from build123d import *

# Parameters (mm, degrees)
CROQUIS1_R              = 3.4
SALIENTE_EXTRUIR1_DEPTH = 360


with BuildPart() as part:
    # Croquis1 → Saliente-Extruir1 (new body)
    with BuildSketch(Plane.XY):
        with BuildLine():
            Line((-4.433640906, 1.227432273), (-4.433640906, 9.707432273))
            Line((-4.433640906, 9.707432273), (1.236359094, 15.377432273))
            Line((1.236359094, 15.377432273), (4.426359094, 15.377432273))
            Line((4.426359094, 15.377432273), (4.426359094, 11.197432273))
            Line((4.426359094, 11.197432273), (5.426359094, 11.197432273))
            ThreePointArc((5.426359094, 11.197432273), (6.133465875, 11.490325492), (6.426359094, 12.197432273))
            Line((6.426359094, 12.197432273), (6.426359094, 19.627432273))
            ThreePointArc((6.426359094, 19.627432273), (5.694126047, 21.395199226), (3.926359094, 22.127432273))
            Line((3.926359094, 22.127432273), (-3.503640906, 22.127432273))
            ThreePointArc((-3.503640906, 22.127432273), (-4.210747688, 21.834539054), (-4.503640906, 21.127432273))
            Line((-4.503640906, 21.127432273), (-4.503640906, 20.127432273))
            Line((-4.503640906, 20.127432273), (-0.323640906, 20.127432273))
            Line((-0.323640906, 20.127432273), (-0.323640906, 16.937432273))
            Line((-0.323640906, 16.937432273), (-5.993640906, 11.267432273))
            Line((-5.993640906, 11.267432273), (-14.473640906, 11.267432273))
            Line((-14.473640906, 11.267432273), (-20.143640906, 16.937432273))
            Line((-20.143640906, 16.937432273), (-20.143640906, 20.127432273))
            Line((-20.143640906, 20.127432273), (-15.963640906, 20.127432273))
            Line((-15.963640906, 20.127432273), (-15.963640906, 21.127432273))
            ThreePointArc((-15.963640906, 21.127432273), (-16.256534125, 21.834539054), (-16.963640906, 22.127432273))
            Line((-16.963640906, 22.127432273), (-24.393640906, 22.127432273))
            ThreePointArc((-24.393640906, 22.127432273), (-26.161407859, 21.395199226), (-26.893640906, 19.627432273))
            Line((-26.893640906, 19.627432273), (-26.893640906, 12.197432273))
            ThreePointArc((-26.893640906, 12.197432273), (-26.600747688, 11.490325492), (-25.893640906, 11.197432273))
            Line((-25.893640906, 11.197432273), (-24.893640906, 11.197432273))
            Line((-24.893640906, 11.197432273), (-24.893640906, 15.377432273))
            Line((-24.893640906, 15.377432273), (-21.703640906, 15.377432273))
            Line((-21.703640906, 15.377432273), (-16.033640906, 9.707432273))
            Line((-16.033640906, 9.707432273), (-16.033640906, 1.227432273))
            Line((-16.033640906, 1.227432273), (-21.703640906, -4.442567727))
            Line((-21.703640906, -4.442567727), (-24.893640906, -4.442567727))
            Line((-24.893640906, -4.442567727), (-24.893640906, -0.262567727))
            Line((-24.893640906, -0.262567727), (-25.893640906, -0.262567727))
            ThreePointArc((-25.893640906, -0.262567727), (-26.600747688, -0.555460946), (-26.893640906, -1.262567727))
            Line((-26.893640906, -1.262567727), (-26.893640906, -8.692567727))
            ThreePointArc((-26.893640906, -8.692567727), (-26.161407859, -10.46033468), (-24.393640906, -11.192567727))
            Line((-24.393640906, -11.192567727), (-16.963640906, -11.192567727))
            ThreePointArc((-16.963640906, -11.192567727), (-16.256534125, -10.899674508), (-15.963640906, -10.192567727))
            Line((-15.963640906, -10.192567727), (-15.963640906, -9.192567727))
            Line((-15.963640906, -9.192567727), (-20.143640906, -9.192567727))
            Line((-20.143640906, -9.192567727), (-20.143640906, -6.002567727))
            Line((-20.143640906, -6.002567727), (-14.473640906, -0.332567727))
            Line((-14.473640906, -0.332567727), (-5.993640906, -0.332567727))
            Line((-5.993640906, -0.332567727), (-0.323640906, -6.002567727))
            Line((-0.323640906, -6.002567727), (-0.323640906, -9.192567727))
            Line((-0.323640906, -9.192567727), (-4.503640906, -9.192567727))
            Line((-4.503640906, -9.192567727), (-4.503640906, -10.192567727))
            ThreePointArc((-4.503640906, -10.192567727), (-4.210747688, -10.899674508), (-3.503640906, -11.192567727))
            Line((-3.503640906, -11.192567727), (3.926359094, -11.192567727))
            ThreePointArc((3.926359094, -11.192567727), (5.694126047, -10.46033468), (6.426359094, -8.692567727))
            Line((6.426359094, -8.692567727), (6.426359094, -1.262567727))
            ThreePointArc((6.426359094, -1.262567727), (6.133465875, -0.555460946), (5.426359094, -0.262567727))
            Line((5.426359094, -0.262567727), (4.426359094, -0.262567727))
            Line((4.426359094, -0.262567727), (4.426359094, -4.442567727))
            Line((4.426359094, -4.442567727), (1.236359094, -4.442567727))
            Line((1.236359094, -4.442567727), (-4.433640906, 1.227432273))
        make_face()
        with Locations(Location((-10.233640906, 5.467432273, 0), (0, 0, 180))):
            Circle(CROQUIS1_R, mode=Mode.SUBTRACT)
        with BuildLine():
            Line((1.417854227, 20.368927407), (4.167854227, 20.368927407))
            ThreePointArc((4.167854227, 20.368927407), (4.521407618, 20.222480798), (4.667854227, 19.868927407))
            Line((4.667854227, 19.868927407), (4.667854227, 17.118927407))
            ThreePointArc((4.667854227, 17.118927407), (4.521407618, 16.765374016), (4.167854227, 16.618927407))
            Line((4.167854227, 16.618927407), (1.417854227, 16.618927407))
            ThreePointArc((1.417854227, 16.618927407), (1.064300837, 16.765374016), (0.917854227, 17.118927407))
            Line((0.917854227, 17.118927407), (0.917854227, 19.868927407))
            ThreePointArc((0.917854227, 19.868927407), (1.064300837, 20.222480798), (1.417854227, 20.368927407))
        make_face(mode=Mode.SUBTRACT)
        with BuildLine():
            Line((-25.13513604, 19.868927407), (-25.13513604, 17.118927407))
            ThreePointArc((-25.13513604, 17.118927407), (-24.988689431, 16.765374016), (-24.63513604, 16.618927407))
            Line((-24.63513604, 16.618927407), (-21.88513604, 16.618927407))
            ThreePointArc((-21.88513604, 16.618927407), (-21.531582649, 16.765374016), (-21.38513604, 17.118927407))
            Line((-21.38513604, 17.118927407), (-21.38513604, 19.868927407))
            ThreePointArc((-21.38513604, 19.868927407), (-21.531582649, 20.222480798), (-21.88513604, 20.368927407))
            Line((-21.88513604, 20.368927407), (-24.63513604, 20.368927407))
            ThreePointArc((-24.63513604, 20.368927407), (-24.988689431, 20.222480798), (-25.13513604, 19.868927407))
        make_face(mode=Mode.SUBTRACT)
        with BuildLine():
            Line((-21.88513604, -9.43406286), (-24.63513604, -9.43406286))
            ThreePointArc((-24.63513604, -9.43406286), (-24.988689431, -9.287616251), (-25.13513604, -8.93406286))
            Line((-25.13513604, -8.93406286), (-25.13513604, -6.18406286))
            ThreePointArc((-25.13513604, -6.18406286), (-24.988689431, -5.83050947), (-24.63513604, -5.68406286))
            Line((-24.63513604, -5.68406286), (-21.88513604, -5.68406286))
            ThreePointArc((-21.88513604, -5.68406286), (-21.531582649, -5.83050947), (-21.38513604, -6.18406286))
            Line((-21.38513604, -6.18406286), (-21.38513604, -8.93406286))
            ThreePointArc((-21.38513604, -8.93406286), (-21.531582649, -9.287616251), (-21.88513604, -9.43406286))
        make_face(mode=Mode.SUBTRACT)
        with BuildLine():
            Line((4.667854227, -8.93406286), (4.667854227, -6.18406286))
            ThreePointArc((4.667854227, -6.18406286), (4.521407618, -5.83050947), (4.167854227, -5.68406286))
            Line((4.167854227, -5.68406286), (1.417854227, -5.68406286))
            ThreePointArc((1.417854227, -5.68406286), (1.064300837, -5.83050947), (0.917854227, -6.18406286))
            Line((0.917854227, -6.18406286), (0.917854227, -8.93406286))
            ThreePointArc((0.917854227, -8.93406286), (1.064300837, -9.287616251), (1.417854227, -9.43406286))
            Line((1.417854227, -9.43406286), (4.167854227, -9.43406286))
            ThreePointArc((4.167854227, -9.43406286), (4.521407618, -9.287616251), (4.667854227, -8.93406286))
        make_face(mode=Mode.SUBTRACT)
    extrude(amount=SALIENTE_EXTRUIR1_DEPTH)


solid = part.part
Geometry: final body of the model. Coordinates: model frame, mm. A direction names the side the tool comes from. Round coordinates to 2 decimals unless told otherwise and drop trailing zeros. Put each result on its own line as item: value. Start each with the question number.
(1) Set-up query: faces 1 (the face through (-10, -0.333, 177)), 2 (the face through (0, 22.127, 177)), 3 (the face through (-17.269, 14.063, 177.48)). Return all of +Z, -Z, +X, -X, +Y, -Y with unobstructed straight access to the full face (end or side cutting, diameter ignored); none if empty.
(2) Section query A-A (z = 198.5). State how many separate pieces and enclosed holes the cut face has, then the cut area to 3 significant figures.
(3) Draft query along X for faces 4 (the face through (-18.908, 12.582, 177.48)), 5 (the face through (-21, -11.193, 177)), 6 (the face through (-16.034, 6, 177)). Return one class per face: +X half, -X half, draft (parallel to the pull), parting line (faces both ways), or undercut.
(4) Contact query for flat-ended pins moving along their axis: pin 1 Ø4 at (y, z) = (4.5, 258) entering from -X; pin 2 Ø4 at (x, z) = (-7, 309.5) entering from +Y; pin 3 Ø0.5 at (y, z) = (-10, 226.5) entering from +X; pin 4 Ø2 at (x, z) = (-16.5, 52) entering from -Y. Output: stop coordinate, or through.
(5) Material intervals for line 1 along X through (y, z) = (-6, 93); line 2 along Y through (x, z) = (2, 172.5); line 3 along X through (y, z) = (19, 308), sorted ascending. Write a range as [from, to].
Findings below:
1. face 1: +Z, -Z, -Y
1. face 2: +Z, -Z, +X, -X, +Y
1. face 3: +Z, -Z
2. separate pieces: 1
2. enclosed holes: 5
2. area: 346 mm2
3. face 4: undercut
3. face 5: draft
3. face 6: -X half
4. pin 1: stops at x = -16.03
4. pin 2: stops at y = 12.26
4. pin 3: stops at x = 6.19
4. pin 4: stops at y = -11.19
5. line 1: x = [-26.89, -25.1], [-21.42, -20.14], [-0.33, 0.95], [4.63, 6.43]
5. line 2: y = [-11.19, -9.43], [-5.68, -4.44], [15.38, 16.62], [20.37, 22.13]
5. line 3: x = [-26.89, -25.14], [-21.39, -20.14], [-0.32, 0.92], [4.67, 6.43]
